from build123d import *

# Parameters (mm, degrees)
SKETCH_3_W                  = 170
SKETCH_3_H                  = 78
SKETCH_3_R                  = 2.75
SKETCH_3_R_2                = 2.25
EXTRUDE_1_DEPTH             = 5
HOLE_WIZARD_M5_1_AT_2_COUNT = 2
HOLE_WIZARD_M5_1_AT_2_PITCH = 13
HOLE_WIZARD_M5_1_AT_3_COUNT = 2
HOLE_WIZARD_M5_1_AT_3_PITCH = 30
HOLE_WIZARD_M5_1_AT_4_COUNT = 2
HOLE_WIZARD_M5_1_AT_4_PITCH = 43
PATTERN_LINEAR_1_COUNT      = 2
PATTERN_LINEAR_1_PITCH      = 36.9
PATTERN_LINEAR_2_COUNT      = 2
PATTERN_LINEAR_2_PITCH      = 156.3


with BuildPart() as part:
    # 草图3 → 凸台-拉伸1 (new body)
    with BuildSketch(Plane.XY):
        with Locations((-85, 39)):
            Rectangle(SKETCH_3_W, SKETCH_3_H)
        with Locations((-140, 68)):
            Circle(SKETCH_3_R, mode=Mode.SUBTRACT)
        with Locations((-140, 10)):
            Circle(SKETCH_3_R, mode=Mode.SUBTRACT)
        with Locations((-50, 10)):
            Circle(SKETCH_3_R, mode=Mode.SUBTRACT)
        with Locations((-50, 68)):
            Circle(SKETCH_3_R, mode=Mode.SUBTRACT)
        with Locations((-104.6634, 40)):
            Circle(SKETCH_3_R_2, mode=Mode.SUBTRACT)
        with Locations((-26.7334, 40)):
            Circle(SKETCH_3_R_2, mode=Mode.SUBTRACT)
    extrude(amount=EXTRUDE_1_DEPTH)

    # 草图6 → M5 螺纹孔1 (revolve, cut)
    with BuildSketch(Plane(origin=(-162.3, 54, 5), x_dir=(0, -1, 0), z_dir=(1, 0, 0))):
        Polygon((0, 0), (0, 13.6618073), (2.1, 12.4), (2.1, 0), align=None)
    hole_wizard_m5_1 = revolve(axis=Axis((-162.3, 54, 11.35), (0, 0, -1)), mode=Mode.SUBTRACT)

    # M5 螺纹孔1 at 2: M5 螺纹孔1 ×2
    with Locations(*[(0, i * HOLE_WIZARD_M5_1_AT_2_PITCH, 0) for i in range(1, HOLE_WIZARD_M5_1_AT_2_COUNT)]):
        add(hole_wizard_m5_1, mode=Mode.SUBTRACT)

    # M5 螺纹孔1 at 3: M5 螺纹孔1 ×2
    with Locations(*[(0, -i * HOLE_WIZARD_M5_1_AT_3_PITCH, 0) for i in range(1, HOLE_WIZARD_M5_1_AT_3_COUNT)]):
        add(hole_wizard_m5_1, mode=Mode.SUBTRACT)

    # M5 螺纹孔1 at 4: M5 螺纹孔1 ×2
    with Locations(*[(0, -i * HOLE_WIZARD_M5_1_AT_4_PITCH, 0) for i in range(1, HOLE_WIZARD_M5_1_AT_4_COUNT)]):
        add(hole_wizard_m5_1, mode=Mode.SUBTRACT)

    # 阵列(线性)1: M5 螺纹孔1 ×2
    with Locations(*[(i * PATTERN_LINEAR_1_PITCH, 0, 0) for i in range(1, PATTERN_LINEAR_1_COUNT)]):
        add(hole_wizard_m5_1, mode=Mode.SUBTRACT)

    # 阵列(线性)1 copy 1 sketch → 阵列(线性)1 copy 1 (revolve, cut)
    with BuildSketch(Plane(origin=(-125.4, 67, 5), x_dir=(0, -1, 0), z_dir=(1, 0, 0))):
        Polygon((0, 0), (0, 13.6618073), (2.1, 12.4), (2.1, 0), align=None)
    revolve(axis=Axis((-125.4, 67, 11.35), (0, 0, -1)), mode=Mode.SUBTRACT)

    # 阵列(线性)1 copy 2 sketch → 阵列(线性)1 copy 2 (revolve, cut)
    with BuildSketch(Plane(origin=(-125.4, 24, 5), x_dir=(0, -1, 0), z_dir=(1, 0, 0))):
        Polygon((0, 0), (0, 13.6618073), (2.1, 12.4), (2.1, 0), align=None)
    revolve(axis=Axis((-125.4, 24, 11.35), (0, 0, -1)), mode=Mode.SUBTRACT)

    # 阵列(线性)1 copy 3 sketch → 阵列(线性)1 copy 3 (revolve, cut)
    with BuildSketch(Plane(origin=(-125.4, 11, 5), x_dir=(0, -1, 0), z_dir=(1, 0, 0))):
        Polygon((0, 0), (0, 13.6618073), (2.1, 12.4), (2.1, 0), align=None)
    revolve(axis=Axis((-125.4, 11, 11.35), (0, 0, -1)), mode=Mode.SUBTRACT)

    # 阵列(线性)2: M5 螺纹孔1 ×2
    with Locations(*[(i * PATTERN_LINEAR_2_PITCH, 0, 0) for i in range(1, PATTERN_LINEAR_2_COUNT)]):
        add(hole_wizard_m5_1, mode=Mode.SUBTRACT)

    # 阵列(线性)2 copy 1 sketch → 阵列(线性)2 copy 1 (revolve, cut)
    with BuildSketch(Plane(origin=(-6, 67, 5), x_dir=(0, -1, 0), z_dir=(1, 0, 0))):
        Polygon((0, 0), (0, 13.6618073), (2.1, 12.4), (2.1, 0), align=None)
    revolve(axis=Axis((-6, 67, 11.35), (0, 0, -1)), mode=Mode.SUBTRACT)

    # 阵列(线性)2 copy 2 sketch → 阵列(线性)2 copy 2 (revolve, cut)
    with BuildSketch(Plane(origin=(-6, 24, 5), x_dir=(0, -1, 0), z_dir=(1, 0, 0))):
        Polygon((0, 0), (0, 13.6618073), (2.1, 12.4), (2.1, 0), align=None)
    revolve(axis=Axis((-6, 24, 11.35), (0, 0, -1)), mode=Mode.SUBTRACT)

    # 阵列(线性)2 copy 3 sketch → 阵列(线性)2 copy 3 (revolve, cut)
    with BuildSketch(Plane(origin=(-6, 11, 5), x_dir=(0, -1, 0), z_dir=(1, 0, 0))):
        Polygon((0, 0), (0, 13.6618073), (2.1, 12.4), (2.1, 0), align=None)
    revolve(axis=Axis((-6, 11, 11.35), (0, 0, -1)), mode=Mode.SUBTRACT)


solid = part.part
Build history of the part. All positions in model axes, mm. Give positions to 0.01 mm unless a question says otherwise; leave off trailing zeros. Order: outer loops, then holes, each group sorted by start corner. A loop starts at its lowest first (then second) coordinate and runs counter-clockwise, first axis right, second up. Notation, with made-up numbers: M -7.5,10 L 39.5,10 A12 ccw 39.5,30 Z; hole C -22.5,48.25 d8. An arc over 180 degrees is marked long. Use one line per item in the form item = value.
Q1. Wall check: probe 1 along X at (y, z) = (54, 1.2); probe 2 along Y at (x, z) = (-6, 3.5); probe 3 along Y at (x, z) = (-140, 3.85). Give the ranges that are in metal, low to high.
Conclusion:
probe_1 = -170 to -164.4, -160.2 to -127.5, -123.3 to -8.1, -3.9 to 0
probe_2 = 0 to 8.9, 13.1 to 21.9, 26.1 to 51.9, 56.1 to 64.9, 69.1 to 78
probe_3 = 0 to 7.25, 12.75 to 65.25, 70.75 to 78
Q2. Pull direction X, two halves, no side cores. Call faces 1 (the cylindrical face through (-137.38, 10.83, 2.46)), 2 (the cylindrical face through (-52.747, 10.121, 2.465)), 3 (the flat face through (0, 38, 2)), 4 (the flat face through (-86, 40, 0)): released by +X, released by -X, zero draft, split by the parting line, or undercut.
Conclusion:
face_1 = undercut
face_2 = undercut
face_3 = released by +X
face_4 = zero draft
Q3. Slice it at C-C, the plane x = -140. Write the cut outline in (y, z), and give its area (3 significant figures).
Conclusion:
outline = M 0,0 L 7.25,0 L 7.25,5 L 0,5 Z; M 12.75,0 L 65.25,0 L 65.25,5 L 12.75,5 Z; M 70.75,0 L 78,0 L 78,5 L 70.75,5 Z
area = 335 mm2
Q4. Slice it at A-A, the plane x = -6. Write the cut outline in (y, z).
Conclusion:
outline = M 0,0 L 8.9,0 L 8.9,5 L 0,5 Z; M 13.1,0 L 21.9,0 L 21.9,5 L 13.1,5 Z; M 26.1,0 L 51.9,0 L 51.9,5 L 26.1,5 Z; M 56.1,0 L 64.9,0 L 64.9,5 L 56.1,5 Z; M 69.1,0 L 78,0 L 78,5 L 69.1,5 Z
Q5. Slice it at D-D, the plane y = 54. Write the cut outline in (x, z), and give its area (3 significant figures).
Conclusion:
outline = M -170,0 L -164.4,0 L -164.4,5 L -170,5 Z; M -160.2,0 L -127.5,0 L -127.5,5 L -160.2,5 Z; M -123.3,0 L -8.1,0 L -8.1,5 L -123.3,5 Z; M -3.9,0 L 0,0 L 0,5 L -3.9,5 Z
area = 787 mm2
Q6. Pin check, flat tip, straight feed: P1, Ø3.5, axis at x = -162.3, y = 67, coming from the -Z side. Stop position of the tip, or through.
Conclusion:
P1 = through
Q7. Slice it at B-B, the plane y = 40. Write the cut outline in (x, z), and give its area (3 significant figures).
Conclusion:
outline = M -170,0 L -106.91,0 L -106.91,5 L -170,5 Z; M -102.41,0 L -28.98,0 L -28.98,5 L -102.41,5 Z; M -24.48,0 L 0,0 L 0,5 L -24.48,5 Z
area = 805 mm2
